Job drawing, mm, ordinate dimensions from the low corner. One solid piece. Coordinates: 2 decimals unless noted, no trailing zeros. Order: outer loops, then holes, each group sorted by start corner. A loop starts at its lowest first (then second) coordinate and runs counter-clockwise, first axis right, second up. Notation, with made-up numbers: (41, 0.5) - (45, 0.5) arc R32 ccw to (45, 32.5) - close; hole circle Ø8 at (2, -37.75). An arc over 180 degrees is marked (long way). Return JSON: item names as keys, results as strings.
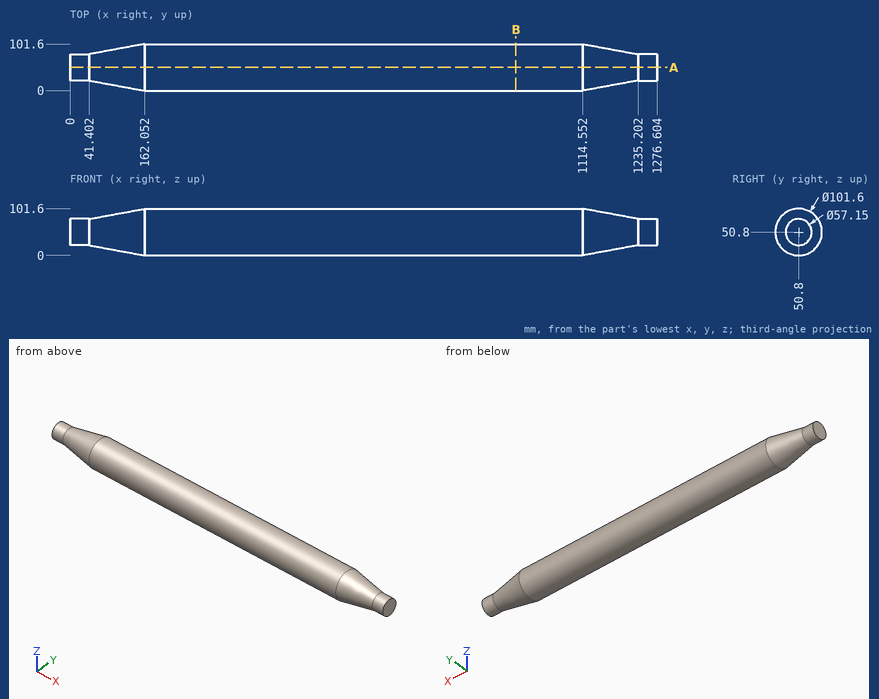
1. Drop flat-ended pins along their axis: pin 1 (5 mm diameter, centred on x = 348, y = 32, fed in from -Z); pin 2 (3 mm diameter, centred on x = 273.5, y = 19, fed in from -Z); pin 3 (5 mm diameter, centred on x = 575, y = 77, fed in from +Z). Give the stop position or say it passes through.
Check values:
{"pin 1": "z = 2.69", "pin 2": "z = 10.03", "pin 3": "z = 95.73"}
2. Probe L1, parallel to Z at x = 732, y = 32; L2, parallel to Y at x = 637, z = 15.5; L3, parallel to Z at x = 1038.5, y = 44.5. List the from-to ranges inside material, lowest first.
Check values:
{"L1": "3.61 to 97.99", "L2": "14.27 to 87.33", "L3": "0.39 to 101.21"}
3. Cut at B-B on x = 969. Give the cut face in (y, z), plus the area to 3 significant figures.
Check values:
{"outline": "circle Ø101.6 at (50.8, 50.8)", "area": "8,110 mm²"}
4. Cut at A-A on y = 50.8. Give the cut face in (x, z) (3 decimals).
Check values:
{"outline": "(0, 22.225) - (41.402, 22.225) - (162.052, 0) - (1114.552, 0) - (1235.202, 22.225) - (1276.604, 22.225) - (1276.604, 79.375) - (1235.202, 79.375) - (1114.552, 101.6) - (162.052, 101.6) - (41.402, 79.375) - (0, 79.375) - close"}
